Drawing for the job (mm, zero at the part's lowest x, y, z). Coordinates: 2 decimals unless noted, no trailing zeros. Write each loop counter-clockwise with the first axis right and the second up, starting at its lowest first coordinate (ties: lowest second). Pieces come first, ordered by that corner, then holes. Notation, with made-up numbers: (59.5, -31.75) - (91.5, -31.75) arc R13 cw to (91.5, -17.75) - close; hole circle Ø1 at (68, 68.5). An arc over 180 degrees is marked (long way). Write each question's results on one line, items separated by ' | '.
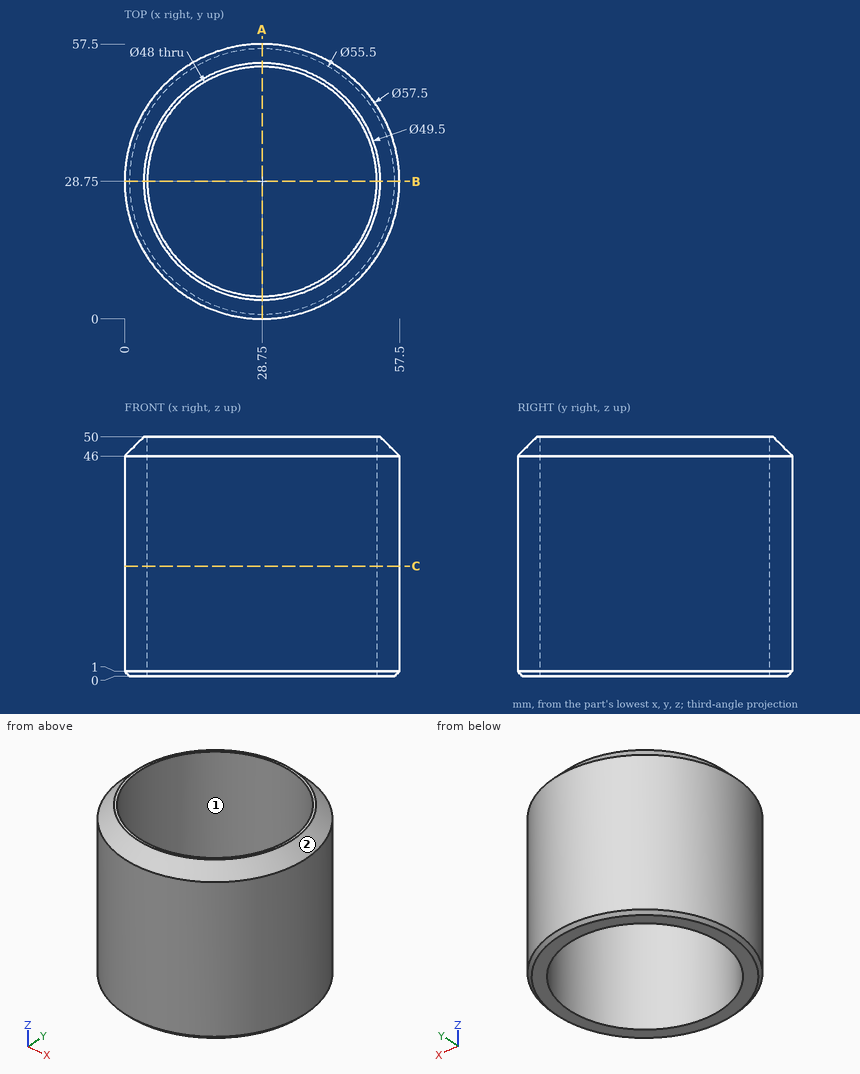
(1) Wall check: line 1 (Y direction, x = 28, z = 37); line 2 (X direction, y = 31.5, z = 28); line 3 (X direction, y = 24.5, z = 13). Give the ranges that are in metal, low to high. Write a range as from..to.
Return value:
line 1: y = 0.01..4.76, 52.74..57.49 | line 2: x = 0.13..4.91, 52.59..57.37 | line 3: x = 0.32..5.13, 52.37..57.18
(2) Saw through at C-C on z = 23. Write the cut outline in (x, y).
Return value:
outline: circle Ø57.5 at (28.75, 28.75); hole circle Ø48 at (28.75, 28.75)
(3) Two-plate mould, pull along X, no slides. Class the marked faces 1 and 2: released by +X, released by -X, zero draft, split by the parting line, or undercut.
Return value:
face 1: undercut | face 2: split by the parting line
(4) Flat gauge pins, fed straight in: P1, Ø2, axis at y = 41.5, z = 26, coming from the -X side; P2, Ø2, axis at x = 42, z = 43, coming from the -Y side; P3, Ø12, axis at x = 15, y = 20, coming from the -Z side; P4, Ø3, axis at x = 50, z = 12, coming from the +Y side. Where does each tip first touch, or does it go through?
Return value:
P1: stops at x = 2.51 | P2: stops at y = 2.74 | P3: passes through | P4: stops at y = 49.64
(5) Saw through at A-A on x = 28.75. Write the cut outline in (y, z).
Return value:
outline: (0, 1) - (1, 0) - (4.75, 0) - (4.75, 50) - (4, 50) - (0, 46) - close; (52.75, 0) - (56.5, 0) - (57.5, 1) - (57.5, 46) - (53.5, 50) - (52.75, 50) - close
